Read the model definition and answer for the solid it produces. Units are mm, in the model's axes. Face numbers are marked on the shaded views. Round coordinates to 2 decimals unless told otherwise and drop trailing zeros. Write each loop counter-clockwise with the first axis right and the second up, starting at its lowest first coordinate (ties: lowest second). Pieces come first, ordered by that corner, then holes. Notation, with made-up numbers: (-24.5, 2.25) - (5.5, 2.25) arc R21 cw to (5.5, 22.25) - close; hole circle Ø2 at (77, -6). An arc over 180 degrees is marked (long way). One line per item, written item: value. Start each with the question number.
(1) Flat-ended cylindrical pins translate along their axes: pin 1 Ø1 at (y, z) = (4, -0.5) entering from -X; pin 2 Ø6 at (x, z) = (-27, 1) entering from -Y; pin 3 Ø5 at (x, z) = (45.5, -1.5) entering from +Y. Find the tip coordinate at first contact, or state that the pin passes through.
(2) A cutting plane is placed at B-B, the plane x = 46. Determine the outline of the cut face in (y, z), plus the area to 3 significant figures.
(3) A cutting plane is placed at C-C, the plane z = 3.5. Determine the outline of the cut face in (x, y).
(4) Find the intervals of material crossed by L1, parallel to Z at x = 46, y = 29.95; L2, parallel to X at y = 27.7, z = 0; L3, parallel to Y at x = 22, z = 4.5, in increasing order.
(5) A cutting plane is placed at D-D, the plane y = -11.5. Determine the outline of the cut face in (x, z).
(6) A cutting plane is placed at A-A, the plane y = -46. Determine the outline of the cut face in (x, z).
(7) The mould has two halves that part along Y. Classify the marked faces 1, 2 and 3: +Y half, -Y half, draft (parallel to the pull), parting line (faces both ways), or undercut.
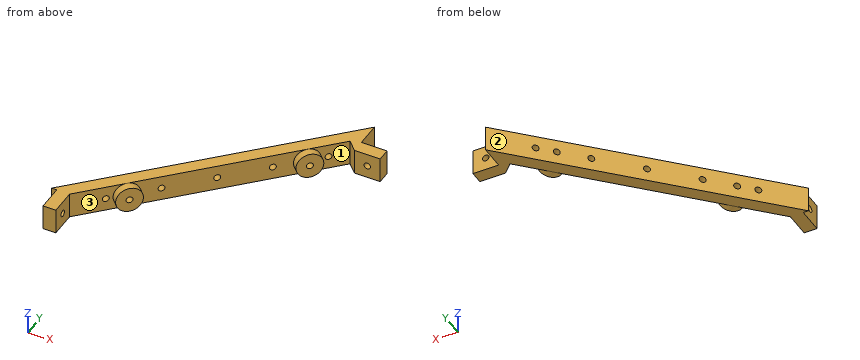
from build123d import *

# Parameters (mm, degrees)
MAIN_DEPTH         = 5
SKETCH2_R          = 1.25
FIXHOLE1_DEPTH     = 83
SKETCH3_R          = 1.25
FIXHOLE2_DEPTH     = 83.5
SKETCH7_R          = 5
BOARDSUPPORT_DEPTH = 3
SKETCH8_R          = 1.25
HOLEFIX_DEPTH      = 66.932503526
SKETCH6_R          = 1.25
CUT_EXTRUDE2_DEPTH = 63.932503526
LPATTERN1_COUNT    = 5
LPATTERN1_PITCH    = 20


with BuildPart() as part:
    # Sketch1 → Main (new body, symmetric)
    with BuildSketch(Plane.XY):
        Polygon((-41, -41), (41, 41), (41, 31.5), (51, 31.5), (51, 26.5), (41, 26.5), (37.25, 30.25), (-34, -41), (-34, -51), (-39, -51), (-39, -41), align=None)
    extrude(amount=MAIN_DEPTH, both=True)

    # Sketch2 → FixHole1 (cut, through all)
    with BuildSketch(Plane(origin=(41, 0, 0), x_dir=(0, 0, -1), z_dir=(1, 0, 0))):
        with Locations((0, -46)):
            Circle(SKETCH2_R)
    extrude(amount=-FIXHOLE1_DEPTH, mode=Mode.SUBTRACT)

    # Sketch3 → FixHole2 (cut, through all)
    with BuildSketch(Plane(origin=(0, 31.5, 0), x_dir=(-1, 0, 0), z_dir=(0, -1, 0))):
        with Locations((-46, 0)):
            Circle(SKETCH3_R)
    extrude(amount=FIXHOLE2_DEPTH, mode=Mode.SUBTRACT)

    # Sketch7 → BoardSupport (add)
    with BuildSketch(Plane(origin=(3.5, -3.5, 0), x_dir=(0, 0, 1), z_dir=(-0.707106781, 0.707106781, 0))):
        with Locations((0, -32.4)):
            Circle(SKETCH7_R)
        with Locations((0, 32.4)):
            Circle(SKETCH7_R)
    extrude(amount=-BOARDSUPPORT_DEPTH)

    # Sketch8 → HoleFix (cut, through all)
    with BuildSketch(Plane(origin=(5.621320344, -5.621320344, 0), x_dir=(0, 0, -1), z_dir=(0.707106781, -0.707106781, 0))):
        with Locations((0, 32.4)):
            Circle(SKETCH8_R)
        with Locations((0, -32.4)):
            Circle(SKETCH8_R)
    extrude(amount=-HOLEFIX_DEPTH, mode=Mode.SUBTRACT)

    # Sketch6 → Cut-Extrude2 (cut, through all)
    with BuildSketch(Plane(origin=(3.5, -3.5, 0), x_dir=(0, 0, 1), z_dir=(-0.707106781, 0.707106781, 0))):
        with Locations((0, 40)):
            Circle(SKETCH6_R)
    cut_extrude2 = extrude(amount=CUT_EXTRUDE2_DEPTH, mode=Mode.SUBTRACT)

    # LPattern1: Cut-Extrude2 ×5
    with Locations(*[Vector(-0.707106781, -0.707106781, 0) * (i * LPATTERN1_PITCH) for i in range(1, LPATTERN1_COUNT)]):
        add(cut_extrude2, mode=Mode.SUBTRACT)


solid = part.part
Here are the results:
1. pin 1: x = 3.5
1. pin 2: y = -37
1. pin 3: y = 31.5
2. outline: (26.5, -5) - (31.5, -5) - (31.5, -1.25) - (26.5, -1.25) - close; (26.5, 1.25) - (31.5, 1.25) - (31.5, 5) - (26.5, 5) - close
2. area: 37.5 mm²
3. outline: (-41, -41) - (-39, -41) - (-39, -51) - (-34, -51) - (-34, -41) - (-21.94, -28.94) - (-19.81, -31.06) - (-14.76, -26.01) - (-16.89, -23.89) - (23.89, 16.89) - (26.01, 14.76) - (31.06, 19.81) - (28.94, 21.94) - (37.25, 30.25) - (41, 26.5) - (51, 26.5) - (51, 31.5) - (41, 31.5) - (41, 41) - close
4. L1: -5 to -1.25, 1.25 to 5
4. L2: 30.64 to 34.7, 39.8 to 44.75, 47.25 to 51
4. L3: 15 to 22
5. outline: (-11.5, -5) - (-4.5, -5) - (-4.5, 5) - (-11.5, 5) - close
6. outline: (-39, -5) - (-34, -5) - (-34, -1.25) - (-39, -1.25) - close; (-39, 1.25) - (-34, 1.25) - (-34, 5) - (-39, 5) - close
7. face 1: undercut
7. face 2: +Y half
7. face 3: -Y half
